The listing builds one solid part. Answer for the finished solid, in the listing's coordinates (mm). A direction names the side the tool comes from. Coordinates: 2 decimals unless noted, no trailing zeros. Order: outer loops, then holes, each group sorted by start corner. A loop starts at its lowest first (then second) coordinate and runs counter-clockwise, first axis right, second up. Notation, with made-up numbers: (42, -34) -> (67, -34) arc R32 cw to (67, 2) -> close; hole circle Ø8 at (-36.5, 57). An arc over 180 degrees is marked (long way). Return JSON: item names as keys, results as strings.
from build123d import *

# Parameters (mm, degrees)
SKETCH_2_R        = 2
EXTRUDE_1_DEPTH   = 7
EXTRUDE_1_2_DEPTH = 7
EXTRUDE_1_3_DEPTH = 7
SKETCH_3_R        = 20
SKETCH_3_R_2      = 10
EXTRUDE_2_DEPTH   = 13
FILLET_1_R        = 5
CHAMFER_1_SIZE    = 5
CHAMFER_1_SIZE2   = 0.437443318
CHAMFER_2_SIZE    = 3.464101615
CHAMFER_2_SIZE_2  = 2
CHAMFER_3_SIZE    = 0.5
CHAMFER_4_SIZE    = 0.5
CHAMFER_4_SIZE2   = 0.550031434


with BuildPart() as part:
    # Sketch 2 → Extrude 1 (new body)
    with BuildSketch(Plane(origin=(0, 0, 0), x_dir=(1, 0, 0), z_dir=(0, 1, 0))):
        with BuildLine():
            Line((10, -17.320508076), (20.980762114, -23.660254038))
            ThreePointArc((20.980762114, -23.660254038), (34.641016151, -20), (30.980762114, -6.339745962))
            Line((30.980762114, -6.339745962), (20, 0))
            ThreePointArc((20, 0), (17.320508076, -10), (10, -17.320508076))
        make_face()
        with Locations(Location((25.980762114, -15, 0), (0, 0, 270))):
            Circle(SKETCH_2_R, mode=Mode.SUBTRACT)
    extrude(amount=EXTRUDE_1_DEPTH)



with BuildPart() as body_2:
    # Sketch 2 → Extrude 1 2 (new body)
    with BuildSketch(Plane(origin=(0, 0, 0), x_dir=(1, 0, 0), z_dir=(0, 1, 0))):
        with BuildLine():
            Line((-20.980762114, -23.660254038), (-10, -17.320508076))
            ThreePointArc((-10, -17.320508076), (-17.320508076, -10), (-20, 0))
            Line((-20, 0), (-30.980762114, -6.339745962))
            ThreePointArc((-30.980762114, -6.339745962), (-34.641016151, -20), (-20.980762114, -23.660254038))
        make_face()
        with Locations(Location((-25.980762114, -15, 0), (0, 0, 270))):
            Circle(SKETCH_2_R, mode=Mode.SUBTRACT)
    extrude(amount=EXTRUDE_1_2_DEPTH)


with BuildPart() as body_3:
    # Sketch 2 → Extrude 1 3 (new body)
    with BuildSketch(Plane(origin=(0, 0, 0), x_dir=(1, 0, 0), z_dir=(0, 1, 0))):
        with BuildLine():
            ThreePointArc((-10, 17.320508076), (0, 20), (10, 17.320508076))
            Line((10, 17.320508076), (10, 30))
            ThreePointArc((10, 30), (0, 40), (-10, 30))
            Line((-10, 30), (-10, 17.320508076))
        make_face()
        with Locations(Location((0, 30, 0), (0, 0, 270))):
            Circle(SKETCH_2_R, mode=Mode.SUBTRACT)
    extrude(amount=EXTRUDE_1_3_DEPTH)


with BuildPart() as part_1:
    add(part.part)

    add(body_2.part)  # Extrude 2 merges body 2

    add(body_3.part)  # Extrude 2 merges body 3
    # Sketch 3 → Extrude 2 (add)
    with BuildSketch(Plane.XZ):
        with Locations(Location((0, 0, 0), (0, 0, 270))):
            Circle(SKETCH_3_R)
        with Locations(Location((0, 0, 0), (0, 0, 270))):
            Circle(SKETCH_3_R_2, mode=Mode.SUBTRACT)
    extrude(amount=-EXTRUDE_2_DEPTH)

    # Fillet 1
    fillet_1_edges = [part_1.edges().sort_by_distance(p)[0] for p in [
        (10, 3.5, 17.320508076),
        (20, 3.5, 0),
        (-10, 3.5, 17.320508076),
        (-20, 3.5, 0),
        (-10, 3.5, -17.320508076),
        (10, 3.5, -17.320508076),
    ]]
    fillet(fillet_1_edges, radius=FILLET_1_R)

    # Chamfer 1
    chamfer_1_edges = [part_1.edges().sort_by_distance(p)[0] for p in [
        (0, 13, 20),
    ]]
    chamfer_1_side = [part_1.faces().sort_by_distance(p)[0] for p in [
        (0, 13, 19.434314575),
    ]]
    chamfer(chamfer_1_edges, length=CHAMFER_1_SIZE, length2=CHAMFER_1_SIZE2, reference=chamfer_1_side[0])

    # Chamfer 2
    # the kernel refuses this chamfer: 3.464101615, 2 mm, written as the material it takes off along each edge
    with BuildSketch(Plane(origin=(12.320508076, 7, 18.660254038), x_dir=(0.4999066103111042, 0.01932676561270069, -0.8658636480983676), z_dir=(0.8660254037844386, 0, 0.5000000000000003)), Plane(origin=(10, 7, -20), x_dir=(-0.9998132206222079, 0.01932676561270069, 0), z_dir=(0, 0, -1)), Plane(origin=(-10, 7, -30), x_dir=(0.9998132206222079, 0.01932676561270069, 0), z_dir=(0, 0, 1)), Plane(origin=(30.980762114, 7, 6.339745962), x_dir=(-0.4999066103111044, 0.01932676561270069, 0.8658636480983674), z_dir=(-0.8660254037844385, 0, -0.5000000000000004))) as chamfer_2_piece_1:
        Polygon((CHAMFER_2_SIZE * 0.999813220662, -CHAMFER_2_SIZE * 0.0193267656135), (-CHAMFER_2_SIZE_2 * 0.0193267656127, -CHAMFER_2_SIZE_2 * 0.999813220622), (0, 0), align=None)
    extrude(amount=10, mode=Mode.SUBTRACT)
    with BuildSketch(Plane(origin=(-25.980762114, 7, 15), x_dir=(-0.5000000000000021, 0, -0.8660254037844373), z_dir=(0.8660254037844373, 0, -0.5000000000000021))) as chamfer_2_piece_2:
        Polygon((10 - CHAMFER_2_SIZE_2, 0), (10, -CHAMFER_2_SIZE), (10, 0), align=None)
    revolve(axis=Axis((-25.980762114, 7, 15), (0, 1, 0)), revolution_arc=180, mode=Mode.SUBTRACT)
    with BuildSketch(Plane(origin=(-22.320508076, 7, 1.339745962), x_dir=(0.49916137187689635, 0.05789386240267152, 0.8645728572665669), z_dir=(-0.8660254037844386, 0, 0.5000000000000001)), Plane(origin=(-20.980762114, 7, 23.660254038), x_dir=(-0.4991613718768962, 0.057893862402671505, -0.8645728572665671), z_dir=(0.8660254037844387, 0, -0.49999999999999983))) as chamfer_2_piece_3:
        Polygon((CHAMFER_2_SIZE_2 * 0.998322743754, -CHAMFER_2_SIZE_2 * 0.0578938624027), (-CHAMFER_2_SIZE * 0.057893862405, -CHAMFER_2_SIZE * 0.998322743793), (0, 0), align=None)
    extrude(amount=10, mode=Mode.SUBTRACT)
    with BuildSketch(Plane(origin=(-24.820508076, 7, -2.990381057), x_dir=(-0.10176135112534013, 0, -0.9948088396356083), z_dir=(-0.9948088396356083, 0, 0.10176135112534013))) as chamfer_2_piece_4_section:
        Polygon((5, CHAMFER_2_SIZE), (5 + CHAMFER_2_SIZE_2, 0), (5, 0), align=None)
    chamfer_2_piece_4 = revolve(axis=Axis((-24.820508076, 7, -2.990381057), (0, -1, 0)), revolution_arc=155.840605946, mode=Mode.PRIVATE)
    chamfer_2_piece_4 = chamfer_2_piece_4 - Plane(origin=(0, 5.431561908, 0), x_dir=(0, 0, -1), z_dir=(0, -1, 0)) * Cylinder(20, 28, mode=Mode.PRIVATE)
    add(chamfer_2_piece_4, mode=Mode.SUBTRACT)
    with BuildSketch(Plane(origin=(-9.820508076, 7, 22.990381057), x_dir=(0.8106490514710499, 0, 0.5855323350158272), z_dir=(-0.5855323350158272, 0, 0.8106490514710499))) as chamfer_2_piece_5_section:
        Polygon((5 + CHAMFER_2_SIZE_2, 0), (5, -CHAMFER_2_SIZE), (5, 0), align=None)
    chamfer_2_piece_5 = revolve(axis=Axis((-9.820508076, 7, 22.990381057), (0, 1, 0)), revolution_arc=155.840605946, mode=Mode.PRIVATE)
    chamfer_2_piece_5 = chamfer_2_piece_5 - Plane(origin=(0, 5.431562064, 0), x_dir=(0, 0, -1), z_dir=(0, -1, 0)) * Cylinder(20, 29, mode=Mode.PRIVATE)
    add(chamfer_2_piece_5, mode=Mode.SUBTRACT)
    with BuildSketch(Plane(origin=(0, 7, -30), x_dir=(1, 0, 0), z_dir=(0, 0, 1))) as chamfer_2_piece_6:
        Polygon((10 - CHAMFER_2_SIZE, 0), (10, -CHAMFER_2_SIZE_2), (10, 0), align=None)
    revolve(axis=Axis((0, 7, -30), (0, 1, 0)), revolution_arc=180, mode=Mode.SUBTRACT)
    with BuildSketch(Plane(origin=(25.980762114, 7, 15), x_dir=(-0.4999999999999975, 0, 0.8660254037844399), z_dir=(-0.8660254037844399, 0, -0.4999999999999975))) as chamfer_2_piece_7:
        Polygon((10 - CHAMFER_2_SIZE, 0), (10, -CHAMFER_2_SIZE_2), (10, 0), align=None)
    revolve(axis=Axis((25.980762114, 7, 15), (0, 1, 0)), revolution_arc=180, mode=Mode.SUBTRACT)
    with BuildSketch(Plane(origin=(-15, 7, -20), x_dir=(-0.9124104025964815, 0, 0.40927650461970855), z_dir=(-0.40927650461970855, 0, -0.9124104025964815))) as chamfer_2_piece_8_section:
        Polygon((5 + CHAMFER_2_SIZE, 0), (5, -CHAMFER_2_SIZE_2), (5, 0), align=None)
    chamfer_2_piece_8 = revolve(axis=Axis((-15, 7, -20), (0, 1, 0)), revolution_arc=155.840605946, mode=Mode.PRIVATE)
    chamfer_2_piece_8 = chamfer_2_piece_8 - Plane(origin=(0, 6.05627025, 0), x_dir=(0, 0, -1), z_dir=(0, -1, 0)) * Cylinder(20, 34, mode=Mode.PRIVATE)
    add(chamfer_2_piece_8, mode=Mode.SUBTRACT)
    with BuildSketch(Plane(origin=(9.820508076, 7, 22.990381057), x_dir=(-0.8106490514711084, 0, 0.5855323350157463), z_dir=(0.5855323350157463, 0, 0.8106490514711084))) as chamfer_2_piece_9_section:
        Polygon((5 + CHAMFER_2_SIZE, 0), (5, CHAMFER_2_SIZE_2), (5, 0), align=None)
    chamfer_2_piece_9 = revolve(axis=Axis((9.820508076, 7, 22.990381057), (0, -1, 0)), revolution_arc=155.840605946, mode=Mode.PRIVATE)
    chamfer_2_piece_9 = chamfer_2_piece_9 - Plane(origin=(0, 6.056270332, 0), x_dir=(0, 0, -1), z_dir=(0, -1, 0)) * Cylinder(20, 34, mode=Mode.PRIVATE)
    add(chamfer_2_piece_9, mode=Mode.SUBTRACT)
    with BuildSketch(Plane(origin=(24.820508076, 7, -2.990381057), x_dir=(0.1017613511254389, 0, -0.9948088396355981), z_dir=(0.9948088396355981, 0, 0.1017613511254389))) as chamfer_2_piece_10_section:
        Polygon((5, -CHAMFER_2_SIZE_2), (5 + CHAMFER_2_SIZE, 0), (5, 0), align=None)
    chamfer_2_piece_10 = revolve(axis=Axis((24.820508076, 7, -2.990381057), (0, 1, 0)), revolution_arc=155.840605946, mode=Mode.PRIVATE)
    chamfer_2_piece_10 = chamfer_2_piece_10 - Plane(origin=(0, 6.056270131, 0), x_dir=(0, 0, -1), z_dir=(0, -1, 0)) * Cylinder(20, 34, mode=Mode.PRIVATE)
    add(chamfer_2_piece_10, mode=Mode.SUBTRACT)
    with BuildSketch(Plane(origin=(15, 7, -20), x_dir=(0.9124104025963968, 0, 0.4092765046198976), z_dir=(0.4092765046198976, 0, -0.9124104025963968))) as chamfer_2_piece_11_section:
        Polygon((5 + CHAMFER_2_SIZE, 0), (5, CHAMFER_2_SIZE_2), (5, 0), align=None)
    chamfer_2_piece_11 = revolve(axis=Axis((15, 7, -20), (0, -1, 0)), revolution_arc=155.840605946, mode=Mode.PRIVATE)
    chamfer_2_piece_11 = chamfer_2_piece_11 - Plane(origin=(0, 6.056270339, 0), x_dir=(0, 0, -1), z_dir=(0, -1, 0)) * Cylinder(20, 34, mode=Mode.PRIVATE)
    add(chamfer_2_piece_11, mode=Mode.SUBTRACT)

    # Chamfer 3
    chamfer_3_edges = [part_1.edges().sort_by_distance(p)[0] for p in [
        (-16.650635095, 0, 21.160254038),
        (-34.641016151, 0, 20),
        (-26.650635095, 0, 3.839745962),
        (-10, 0, -25),
        (0, 0, -40),
        (10, 0, -25),
        (-17.320508076, 0, -10),
        (0, 0, 20),
        (17.320508076, 0, -10),
        (-10.527864045, 0, -17.763932023),
        (-20.647948425, 0, -0.235431699),
        (-10.12008438, 0, 17.999363722),
        (10.12008438, 0, 17.999363722),
        (20.647948425, 0, -0.235431699),
        (16.650635095, 0, 21.160254038),
        (10.527864045, 0, -17.763932022),
        (26.650635095, 0, 3.839745962),
        (34.641016151, 0, 20),
    ]]
    chamfer(chamfer_3_edges, length=CHAMFER_3_SIZE)

    # Chamfer 4
    chamfer_4_edges = [part_1.edges().sort_by_distance(p)[0] for p in [
        (0, 12.562556682, 20),
    ]]
    chamfer_4_side = [part_1.faces().sort_by_distance(p)[0] for p in [
        (0, 12.781278341, 17.5),
    ]]
    chamfer(chamfer_4_edges, length=CHAMFER_4_SIZE, length2=CHAMFER_4_SIZE2, reference=chamfer_4_side[0])


solid = part_1.part
1. For faces 1 (the face through (-11.3, 4.86, 17.42)), 2 (the face through (-23, 7, 15)), 3 (the face through (16.713, 0.254, 20.912)), 4 (the face through (-8.244, 6.014, -25.07)), determine the directions among +Z, -Z, +X, -X, +Y, -Y from which every point of the face is accessible in a straight line to the end or side of a thin tool.
Answer block:
{"face 1": "+Z, +Y", "face 2": "+Z, -X, +Y", "face 3": "+Z, -Y", "face 4": "-Z, -X, +Y"}
2. The part is cut by section B-B on x = 0. Give the number of separate pieces and of enclosed holes in the cut face, and give its area (3 significant figures).
Answer block:
{"separate pieces": "3", "enclosed holes": "0", "area": "366 mm2"}
3. Consider line 1 (X direction, y = 5.25, z = 15); line 2 (X direction, y = 1.75, z = -30); line 3 (X direction, y = 5.75, z = 15). Determine where each line is inside the solid, lowest interval first. Write a range as from..to.
Answer block:
{"line 1": "x = -34.99..-27.98, -23.98..23.98, 27.98..35.55", "line 2": "x = -10..-2, 2..10", "line 3": "x = -34.7..-27.98, -23.98..23.98, 27.98..34.68"}
4. Each of these flat-tipped pins is pushed along its axis until it touches: pin 1 Ø10 at (x, z) = (18, 4) entering from +Y; pin 2 Ø9 at (x, z) = (23, 12.5) entering from +Y; pin 3 Ø2 at (x, y) = (-14, 8.5) entering from -Z; pin 4 Ø1.5 at (x, y) = (-6, 2) entering from -Z. Where does it stop, or does it pass through?
Answer block:
{"pin 1": "stops at y = 13", "pin 2": "stops at y = 7", "pin 3": "stops at z = -15.2", "pin 4": "stops at z = -38.51"}
5. The part is cut by section A-A on z = -23.5. Give the vertices of the cut face in (x, y), and give its area (3 significant figures).
Answer block:
{"outline": "(-10, 0.5) -> (-9.5, 0) -> (9.5, 0) -> (10, 0.5) -> (10, 5) -> (6.54, 7) -> (-6.54, 7) -> (-10, 5) -> close", "area": "133 mm2"}
